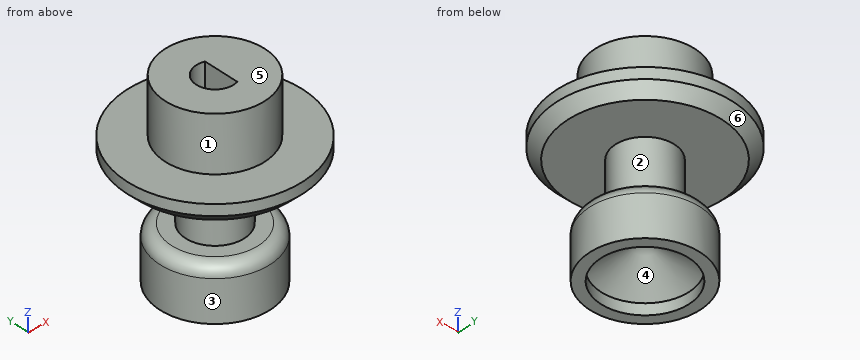
```python
from build123d import *

# Parameters (mm, degrees)
F0_R      = 6.3637373436
F1_DEPTH  = 6.096
F2_R      = 3.4022099148
F3_DEPTH  = 12.7
F5_R      = 10.1544070979
F6_DEPTH  = 2.54
F8_R      = 5.7592976
F9_DEPTH  = 6.35
F12_DEPTH = 6.35
F13_D     = 10.16
F13_DEPTH = 1.27
F13_TIP   = 3.0523719447
F14_R     = 1.3490625387
F15_SIZE  = 1.27


with BuildPart() as f1:
    # F0 (on Top) → F1 (new body)
    with BuildSketch(Plane.XY):
        Circle(F0_R)
    extrude(amount=F1_DEPTH)

    # F2 (on Top) → F3 (join)
    with BuildSketch(Plane.XY):
        Circle(F2_R)
    extrude(amount=F3_DEPTH)

    # F5 (on offset) → F6 (join)
    with BuildSketch(Plane.XY.offset(12.7)):
        Circle(F5_R)
    extrude(amount=F6_DEPTH)

    # F8 (on offset) → F9 (join)
    with BuildSketch(Plane.XY.offset(15.24)):
        Circle(F8_R)
    extrude(amount=F9_DEPTH)

    # F11 (on offset) → F12 (cut)
    with BuildSketch(Plane.XY.offset(21.59)):
        with BuildLine():
            Line((0.7198907698, 0), (0.7198907698, 2.0371562))
            ThreePointArc((0.7198907698, 2.0371562), (-2.1606129, 0), (0.7198907698, -2.0371562))
            Line((0.7198907698, -2.0371562), (0.7198907698, 0))
        make_face()
    extrude(amount=-F12_DEPTH, mode=Mode.SUBTRACT)

    # F13
    with Locations(Plane(origin=(0, 0, 0), x_dir=(1, 0, 0), z_dir=(0, 0, -1))):
        with Locations((0, 0)):
            Hole(F13_D / 2, depth=F13_DEPTH)
            with Locations((0, 0, -(F13_DEPTH + F13_TIP / 2))):  # 118° drill point
                Cone(0, F13_D / 2, F13_TIP, mode=Mode.SUBTRACT)

    # F14
    f14_edges = [f1.edges().sort_by_distance(p)[0] for p in [
        (-6.363737, 0, 6.096),
    ]]
    fillet(f14_edges, radius=F14_R)

    # F15
    f15_edges = [f1.edges().sort_by_distance(p)[0] for p in [
        (-10.154407, 0, 12.7),
    ]]
    chamfer(f15_edges, length=F15_SIZE)


solid = f1.part
```
Could you check a few things on this model? Use its own coordinates, in mm. Face numbers are marked on the shaded views. A direction names the side the tool comes from. Coordinates: 2 decimals unless noted, no trailing zeros. Write each loop counter-clockwise with the first axis right and the second up, starting at its lowest first coordinate (ties: lowest second). Pieces come first, ordered by that corner, then holes. Notation, with made-up numbers: M 62.25,-32.5 L 109.25,-32.5 A4 ccw 109.25,-26.5 Z; hole C 76.5,38 d9. An arc over 180 degrees is marked long. Answer as CSV lines item,"result". Start each with the question number.
1) We'd pull the mould along Y, two halves only. Please class the marked faces 4, 5 and 6: +Y half, -Y half, draft (parallel to the pull), parting line (faces both ways), or undercut.
2) For the marked faces 1, 2 and 3, which set-ups out of +Z, -Z, +X, -X, +Y, -Y let a thin tool reach every point of the face, with its end or its side?
3) Please list where these lines run through material, in increasing order: line 1 (Y direction, x = 0, z = 16.75); line 2 (Y direction, x = 0, z = 0.8); line 3 (Z direction, x = -8.25, y = 1). Write a range as from..to.
4) For P1, Ø1.4, axis at x = -1, y = -1, coming from the +Z side; P2, Ø1.5, axis at y = 0.5, z = 13.5, coming from the -X side; P3, Ø2.5, axis at x = 0, y = 0, coming from the -Z side; P4, Ø1.5, axis at x = 1.5, z = 3, coming from the -Y side, each with a flat end and sliding along its axis, tell me the tip position at first contact or that it passes through.
5) I want a section at A-A, the plane z = 17.5. Please give me the cut outline in (x, y), and give its area (3 significant figures).
6) I want a section at B-B, the plane z = 8. Please give me the cut outline in (x, y), and give its area (3 significant figures).
Data:
1,face 4,"undercut"
1,face 5,"draft"
1,face 6,"parting line"
2,face 1,"+Z"
2,face 2,"none"
2,face 3,"-Z"
3,line 1,"y = -5.76..-2.16, 2.16..5.76"
3,line 2,"y = -6.36..-5.08, 5.08..6.36"
3,line 3,"z = 12.7..15.24"
4,P1,"stops at z = 15.24"
4,P2,"stops at x = -10.15"
4,P3,"stops at z = 3.57"
4,P4,"stops at y = -6.32"
5,outline,"C 0,0 d11.52; hole M 0.72,-2.04 L 0.72,2.04 A2.16 ccw long Z"
5,area,"93.8 mm^2"
6,outline,"C 0,0 d6.8"
6,area,"36.4 mm^2"
